```python
from build123d import *

# Parameters (mm, degrees)
F0_W      = 14.6431
F0_H      = 66.2686
F2_R      = 64.2874
F3_DEPTH  = 21.844
F5_DEPTH  = 66.2696
F6_R      = 1.5748
F7_SIZE   = 0.7874
F10_SIZE2 = 3.65151
F10_SIZE  = 6.3246


with BuildPart() as f1:
    # F0 (on Right) → F1 (revolve)
    with BuildSketch(Plane.YZ):
        with Locations((61.55055, -33.1343)):
            Rectangle(F0_W, F0_H)
    revolve(axis=Axis((0, 0, -33.1343), (0, 0, -1)))

    # F2 (on face) → F3 (cut)
    with BuildSketch(Plane.XY):
        Circle(F2_R)
    extrude(amount=-F3_DEPTH, mode=Mode.SUBTRACT)

    # F4 (on face) → F5 (cut, through all)
    with BuildSketch(Plane(origin=(0, 0, -66.2686), x_dir=(1, 0, 0), z_dir=(0, 0, -1))):
        Polygon((-54.229, 31.309128), (-54.229, -31.309128), (0, -62.618255), (54.229, -31.309128), (54.229, 31.309128), (0, 62.618255), align=None)
    extrude(amount=-F5_DEPTH, mode=Mode.SUBTRACT)

    # F6
    f6_edges = [f1.edges().sort_by_distance(p)[0] for p in [
        (-64.2874, 0, -21.844),
    ]]
    fillet(f6_edges, radius=F6_R)

    # F7
    f7_edges = [f1.edges().sort_by_distance(p)[0] for p in [
        (0, -68.8721, 0),
        (-64.2874, 0, 0),
    ]]
    chamfer(f7_edges, length=F7_SIZE)

    # F8 (on Right) → F9 (revolve, cut)
    with BuildSketch(Plane.YZ):
        Polygon((0, -2.3749), (-63.8937, -66.2686), (0, -66.2686), align=None)
    revolve(axis=Axis((0, 0, -34.32175), (0, 0, 1)), mode=Mode.SUBTRACT)

    # F10
    f10_edges = [f1.edges().sort_by_distance(p)[0] for p in [
        (0, -68.8721, -66.2686),
    ]]
    chamfer(f10_edges, length=F10_SIZE, length2=F10_SIZE2)


solid = f1.part
```
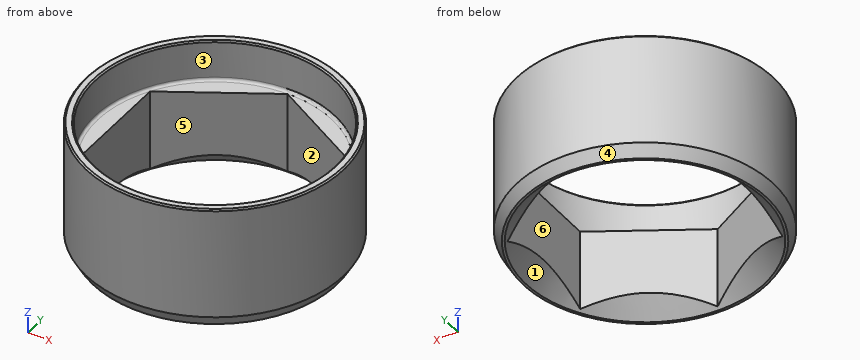
Could you check a few things on this model? Use its own coordinates, in mm. Face numbers are marked on the shaded views. A direction names the side the tool comes from. Give positions to 0.01 mm unless a question says otherwise; leave off trailing zeros. Order: outer loops, then holes, each group sorted by start corner. A loop starts at its lowest first (then second) coordinate and runs counter-clockwise, first axis right, second up.
Q1. I'm going to push flat-ended pins straight in: P1, Ø1, axis at x = -13, z = -16.5, coming from the +Y side; P2, Ø13, axis at y = 3, z = -41.5, coming from the +X side; P3, Ø8, axis at y = -22.5, z = -26, coming from the -X side. Where does each tip first touch, or does it pass through?
Q2. Suppose I cut it at A-A, the plane y = 0. Write out the boundary of the cut face in (x, z).
Q3. For the marked faces 1, 2 and 3, which set-ups out of +Z, -Z, +X, -X, +Y, -Y let a thin tool reach every point of the face, with its end or its side?
Q4. Suppose I cut it at C-C, the plane z = -9.5. Write out the boundary of the cut face in (x, y).
Q5. Suppose I cut it at B-B, the plane z = -33.5. Write out the boundary of the cut face in (x, y), and give its area (3 significant figures).
Q6. If I drill on line 1 along Y through (x, z) = (54, -21); line 2 along Y through (x, z) = (37, -13.5); line 3 along X through (y, z) = (-39, -27.5), over which ranges is the centre line in solid material (lowest first)?
Q7. We'd pull the mould along X, two halves only. Please class the marked faces 4, 5 and 6: +X half, -X half, draft (parallel to the pull), parting line (faces both ways), or undercut.
Solution:
1. P1: stops at y = 67.73
1. P2: stops at x = 68.87
1. P3: stops at x = -66.34
2. outline: (-68.87, -59.94) - (-65.22, -66.27) - (-63.89, -66.27) - (-54.23, -56.6) - (-54.23, -21.84) - (-62.71, -21.84) arc R1.57 cw to (-64.29, -20.27) - (-64.29, -0.79) - (-65.07, 0) - (-68.08, 0) - (-68.87, -0.79) - close; (54.23, -56.6) - (63.89, -66.27) - (65.22, -66.27) - (68.87, -59.94) - (68.87, -0.79) - (68.08, 0) - (65.07, 0) - (64.29, -0.79) - (64.29, -20.27) arc R1.57 cw to (62.71, -21.84) - (54.23, -21.84) - close
3. face 1: -Z
3. face 2: +Z, -Z
3. face 3: +Z
4. outline: circle Ø137.74 at (0, 0); hole circle Ø128.57 at (0, 0)
5. outline: circle Ø137.74 at (0, 0); hole (-54.23, -31.31) - (0, -62.62) - (54.23, -31.31) - (54.23, 31.31) - (0, 62.62) - (-54.23, 31.31) - close
5. area: 4,710 mm2
6. line 1: y = -42.75 to -34.55, 34.55 to 42.75
6. line 2: y = -58.09 to -52.57, 52.57 to 58.09
6. line 3: x = -56.77 to -40.91, 40.91 to 56.77
7. face 4: parting line
7. face 5: undercut
7. face 6: undercut
